```python
from build123d import *

# Parameters (mm, degrees)
BOSS_EXTRUDE1_DEPTH = 3
SKETCH2_W           = 15
SKETCH2_H           = 25
CUT_EXTRUDE1_DEPTH  = 1
SKETCH3_R           = 1
CUT_EXTRUDE2_DEPTH  = 2
SKETCH4_R           = 1
CUT_EXTRUDE4_DEPTH  = 3


with BuildPart() as part:
    # Sketch1 → Boss-Extrude1 (new body)
    with BuildSketch(Plane(origin=(0, 0, 0), x_dir=(1, 0, 0), z_dir=(0, 1, 0))):
        with BuildLine():
            Line((-32.058823529, 17.823529412), (17.941176471, 17.823529412))
            ThreePointArc((17.941176471, 17.823529412), (21.476710377, 16.359063318), (22.941176471, 12.823529412))
            Line((22.941176471, 12.823529412), (22.941176471, -37.176470588))
            ThreePointArc((22.941176471, -37.176470588), (21.476710377, -40.712004494), (17.941176471, -42.176470588))
            Line((17.941176471, -42.176470588), (-32.058823529, -42.176470588))
            ThreePointArc((-32.058823529, -42.176470588), (-35.594357435, -40.712004494), (-37.058823529, -37.176470588))
            Line((-37.058823529, -37.176470588), (-37.058823529, 12.823529412))
            ThreePointArc((-37.058823529, 12.823529412), (-35.594357435, 16.359063318), (-32.058823529, 17.823529412))
        make_face()
    extrude(amount=BOSS_EXTRUDE1_DEPTH)

    # Sketch2 → Cut-Extrude1 (cut)
    with BuildSketch(Plane(origin=(0, 0, 0), x_dir=(1, 0, 0), z_dir=(0, 1, 0))):
        with Locations((-29.558823529, -12.176470588)):
            Rectangle(SKETCH2_W, SKETCH2_H)
        with Locations((15.441176471, -12.176470588)):
            Rectangle(SKETCH2_W, SKETCH2_H)
    extrude(amount=CUT_EXTRUDE1_DEPTH, mode=Mode.SUBTRACT)

    # Sketch3 → Cut-Extrude2 (cut)
    with BuildSketch(Plane(origin=(0, 1, 0), x_dir=(-1, 0, 0), z_dir=(0, -1, 0))):
        with Locations(Location((29.558823529, -20.176470588, 0), (0, 0, 90))):
            Circle(SKETCH3_R)
        with Locations(Location((29.558823529, -4.176470588, 0), (0, 0, 90))):
            Circle(SKETCH3_R)
        with Locations(Location((-15.441176471, -20.176470588, 0), (0, 0, 90))):
            Circle(SKETCH3_R)
        with Locations(Location((-15.441176471, -4.176470588, 0), (0, 0, 90))):
            Circle(SKETCH3_R)
    extrude(amount=-CUT_EXTRUDE2_DEPTH, mode=Mode.SUBTRACT)

    # Sketch4 → Cut-Extrude4 (cut)
    with BuildSketch(Plane(origin=(0, 0, 0), x_dir=(-1, 0, 0), z_dir=(0, -1, 0))):
        with Locations(Location((7.058823529, -12.176470588, 0), (0, 0, 90))):
            Circle(SKETCH4_R)
    extrude(amount=-CUT_EXTRUDE4_DEPTH, mode=Mode.SUBTRACT)


solid = part.part
```
The model under review builds one solid part; all positions refer to its coordinate system, in mm. A direction names the side the tool comes from. Coordinates: 2 decimals unless noted, no trailing zeros. Write each loop counter-clockwise with the first axis right and the second up, starting at its lowest first coordinate (ties: lowest second). Pieces come first, ordered by that corner, then holes. Notation, with made-up numbers: (-3, 33) - (2, 33) arc R36 ccw to (2, 71) - close; hole circle Ø2 at (51.5, -1). An arc over 180 degrees is marked (long way). Answer in a Markdown table with one row per item. Add a question column.
Q1. Consider section A-A on x = -23. Give the boundary of the cut face in (y, z), then the cut area to 3 significant figures.
Q2. Clearance check with flat-ended pins moving along their axes: pin 1 (3 mm diameter, centred on x = 15.44, z = 4.18, fed in from +Y); pin 2 (1.2 mm diameter, centred on x = 15.44, z = 20.18, fed in from -Y); pin 3 (12 mm diameter, centred on x = 16.5, z = 16.5, fed in from -Y). State where each tip first meets the part, or that it passes through.
Q3. To check wall thickness, follow line 1 along X through (y, z) = (2.6, 20); line 2 along X through (y, z) = (2.15, 21); line 3 along X through (y, z) = (2.35, 12). State the ranges of each line that lie inside material, in increasing order. Write a range as from..to.
Q4. Draft analysis for pull direction Z (two halves, no side actions). For faces 1 (the face through (16.284, 1.986, 3.639)), 2 (the face through (-35.555, 1.479, 40.751)), 3 (the face through (-37.059, 2, 13)), state which applies: +Z half, -Z half, draft (parallel to the pull), parting line (faces both ways), or undercut.
Q5. For faces 4 (the face through (-30, 1, 12)), 5 (the face through (-29.94, 1.99, 19.25)), 6 (the face through (15, 1, 12)), list the 3-axis set-ups (+Z, -Z, +X, -X, +Y, -Y) from which the entire face can be reached by the end or side of a thin tool; tool diameter is ignored.
Answers below:
| question | item | result |
|---|---|---|
| 1 | outline | (0, -17.82) - (3, -17.82) - (3, 42.18) - (0, 42.18) - (0, 24.68) - (1, 24.68) - (1, -0.32) - (0, -0.32) - close |
| 1 | area | 155 mm² |
| 2 | pin 1 | y = 3 |
| 2 | pin 2 | through |
| 2 | pin 3 | y = 1 |
| 3 | line 1 | -37.06..-30.54, -28.57..14.46, 16.43..22.94 |
| 3 | line 2 | -37.06..-30.13, -28.99..14.87, 16.01..22.94 |
| 3 | line 3 | -37.06..-8.04, -6.07..22.94 |
| 4 | face 1 | undercut |
| 4 | face 2 | +Z half |
| 4 | face 3 | draft |
| 5 | face 4 | -X, -Y |
| 5 | face 5 | +Y, -Y |
| 5 | face 6 | +X, -Y |
